Build history of the part. All positions in model axes, mm. A direction names the side the tool comes from. Give positions to 0.01 mm unless a question says otherwise; leave off trailing zeros. Write each loop counter-clockwise with the first axis right and the second up, starting at its lowest first coordinate (ties: lowest second). Pieces come first, ordered by that corner, then holes. Notation, with made-up numbers: M 89,54.25 L 138,54.25 A23 ccw 138,72.25 Z; hole C 78,-1 d5. An arc over 180 degrees is marked long. One line per item, written item: value. Start each with the question number.
from build123d import *

# Parameters (mm, degrees)
F1_DEPTH  = 80
F2_W      = 10.1163312793
F2_H      = 100.1585014164
F2_W_2    = 10.3900524974
F3_DEPTH  = 15
F6_W      = 19.9106484652
F6_H      = 22.7042857278
F7_DEPTH  = 17.6
F8_W      = 20.5874107778
F8_H      = 22.7042857278
F9_DEPTH  = 17.7
F10_W     = 46.9934158027
F10_H     = 17.6760927897
F10_H_2   = 21.9856097649
F11_DEPTH = 10.4
F13_DEPTH = 25
F15_DEPTH = 25


# Not quite as in the source:
# - a feature of the source that left no trace in its solid (it failed there, or was rolled back) is left out


with BuildPart() as f1:
    # F0 (on Right) → F1 (new body)
    with BuildSketch(Plane.YZ):
        Polygon((22.4307589233, 109.4066873193), (-17.082426697, 17.6664423198), (0, 17.6664423198), (38.2366999984, 109.4066873193), align=None)
        Polygon((-39.7867124248, 17.6664423198), (-39.2026986647, 0), (49.7872419655, 0), (49.7872419655, 17.6664423198), (0, 17.6664423198), (-17.082426697, 17.6664423198), align=None)
        Polygon((-50.955273211, 17.6664423198), (-50.3712594509, 0), (-39.2026986647, 0), (-39.7867124248, 17.6664423198), align=None)
        Polygon((-50.3712594509, 38.982976228), (-50.955273211, 17.6664423198), (-39.7867124248, 17.6664423198), (-40.4824339626, 38.7120499047), align=None)
    extrude(amount=F1_DEPTH)

    # F2 (on face) → F3 (join)
    with BuildSketch(Plane(origin=(0, 0, 0), x_dir=(1, 0, 0), z_dir=(0, 0, -1))):
        with Locations((5.0581656396, 0.2920087427)):
            Rectangle(F2_W, F2_H)
        with Locations((74.8049737513, 0.2920087427)):
            Rectangle(F2_W_2, F2_H)
    extrude(amount=F3_DEPTH)

    # F6 (on face) → F7 (join)
    with BuildSketch(Plane.XY.offset(17.6664423198)):
        with Locations((39.5665168762, -28.4345695609)):
            Rectangle(F6_W, F6_H)
    extrude(amount=-F7_DEPTH)

    # F8 (on face) → F9 (cut)
    with BuildSketch(Plane.XY.offset(17.6664423198)):
        with Locations((38.6653598398, -28.4345695609)):
            Rectangle(F8_W, F8_H)
    extrude(amount=-F9_DEPTH, mode=Mode.SUBTRACT)

    # F10 (on face) → F11 (cut)
    with BuildSketch(Plane(origin=(0, -50.316272907, -1.6633454095), x_dir=(1, 0, 0), z_dir=(0, -0.9994540383, -0.0330397541))):
        with Locations((39.2467323691, 10.5023004233)):
            Rectangle(F10_W, F10_H)
        with Locations((39.2467323691, 30.3331517006)):
            Rectangle(F10_W, F10_H_2)
    extrude(amount=-F11_DEPTH, mode=Mode.SUBTRACT)

    # F12 (on face) → F13 (cut)
    with BuildSketch(Plane(origin=(0, 0, 0), x_dir=(1, 0, 0), z_dir=(0, 0, -1))):
        Polygon((62.7434402704, 50.3712594509), (15.7500244677, 50.3712594509), (15.7500244677, 40.7608151436), (65.7564029098, 40.7608151436), (65.7564029098, 50.3712594509), align=None)
    extrude(amount=-F13_DEPTH, mode=Mode.SUBTRACT)

    # F14 (on face) → F15 (cut)
    with BuildSketch(Plane(origin=(0, 0, 0), x_dir=(1, 0, 0), z_dir=(0, 0, -1))):
        Polygon((62.1888265014, 40.7608151436), (15.7500244677, 40.7608151436), (15.7500244677, 39.7867124248), (28.3716544509, 39.7867124248), (48.9590652287, 39.7867124248), (62.1888265014, 39.7867124248), align=None)
    extrude(amount=-F15_DEPTH, mode=Mode.SUBTRACT)


solid = f1.part
1) Band-saw the part on A-A (y = -29). List the corners of the cut face in (x, z), then the cut area to 3 significant figures.
2) Mould opens along Y. For faces 5 (the face through (39.44, 18.85, 62.89)), 6 (the face through (64, -28, 17.666)), 7 (the face through (39.44, 2.95, 64.18)), 8 (the face through (39, 25, 17.666)) say: released by +Y, released by -Y, zero draft, split by the parting line, or undercut.
3) Probe line 1 along X through (y, z) = (-4.5, -5.5); line 2 along X through (y, z) = (-20, 16); line 3 along Z through (x, y) = (76, 40). List the from-to ranges inside material, lowest first. Write a range as from..to.
4) Band-saw the part on C-C (z = 20.5). List the corners of the cut face in (x, y).
5) Tool access for faces 1 (the face through (80, -1, 20)), 2 (the face through (5, -50.371, -7)), 3 (the face through (64, -50.371, 12)), 4 (the face through (48.959, -29, 9)): list every direction of +Z, -Z, +X, -X, +Y, -Y with a clear straight run to the whole face (end or side of a thin tool).
6) Drop flat-ended pins along their axis: P1, Ø19.5, axis at x = 34.5, z = 12.5, coming from the -Y side; P2, Ø6, axis at x = 19, z = 31, coming from the +Y side; P3, Ø11.5, axis at x = 43.5, y = -43, coming from the -Z side. Give the stop position or say it passes through.
7) Band-saw the part on D-D (x = 12.5). List the corners of the cut face in (y, z), then the cut area to 3 significant figures.
8) Band-saw the part on B-B (x = 56.5). List the corners of the cut face in (y, z).
Model answer:
1. outline: M 0,-15 L 10.12,-15 L 10.12,0 L 28.37,0 L 28.37,17.67 L 0,17.67 Z; M 48.96,0 L 69.61,0 L 69.61,-15 L 80,-15 L 80,17.67 L 48.96,17.67 Z
1. area: 1,360 mm²
2. face 5: released by +Y
2. face 6: undercut
2. face 7: undercut
2. face 8: zero draft
3. line 1: x = 0..10.12, 69.61..80
3. line 2: x = 0..28.37, 48.96..80
3. line 3: z = -15..17.67
4. outline: M 0,-50.88 L 15.75,-50.88 L 15.75,-39.88 L 0,-39.88 Z; M 0,-15.86 L 80,-15.86 L 80,1.18 L 0,1.18 Z; M 62.19,-40.64 L 62.74,-40.64 L 62.74,-40.76 L 65.76,-40.76 L 65.76,-50.37 L 62.74,-50.37 L 62.74,-50.88 L 80,-50.88 L 80,-39.88 L 62.19,-39.88 Z
5. face 1: +Z, -Z, +X, +Y, -Y
5. face 2: -Z, +X, -X, -Y
5. face 3: -Z
5. face 4: +Z, -Z, -Y
6. P1: stops at y = -39.79
6. P2: stops at y = 6.81
6. P3: stops at z = 25
7. outline: M -50.96,17.67 L -50.37,0 L 49.79,0 L 49.79,17.67 L 0,17.67 L 38.24,109.41 L 22.43,109.41 L -17.08,17.67 L -39.79,17.67 L -40.48,38.71 L -50.37,38.98 Z
7. area: 3,510 mm²
8. outline: M -41.25,38.73 L -40.79,25 L -40.03,25 L -40.48,38.71 Z; M -39.79,0 L 49.79,0 L 49.79,17.67 L 0,17.67 L 38.24,109.41 L 22.43,109.41 L -17.08,17.67 L -39.79,17.67 Z
